Source: CAD feature listing. Evaluate the final solid. Frame: model axes, mm. Give positions to 0.01 mm unless a question says otherwise; leave off trailing zeros. Put each result on its own line as item: value. Start each with the question number.
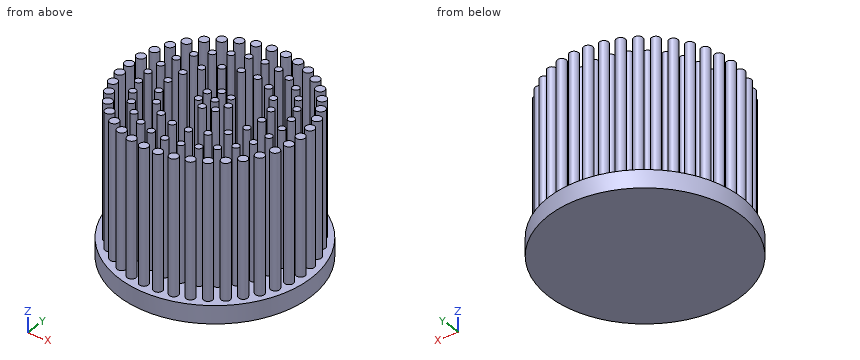
```python
from build123d import *

# Parameters (mm, degrees)
F2_R     = 43
F3_DEPTH = 8
F4_R     = 1.5
F4_R_2   = 2
F5_DEPTH = 60


with BuildPart() as f3:
    # F2 (on Top) → F3 (new body)
    with BuildSketch(Plane.XY):
        Circle(F2_R)
    extrude(amount=F3_DEPTH)

    # F4 (on face) → F5 (join)
    with BuildSketch(Plane.XY.offset(8)):
        Circle(F4_R)
        with Locations((6, 0)):
            Circle(F4_R)
        with Locations((21, 0)):
            Circle(F4_R)
        with Locations((38.41, 0)):
            Circle(F4_R_2)
        with Locations((3.7409388112, 4.6909888948)):
            Circle(F4_R)
        with Locations((-1.3351256037, 5.8495674731)):
            Circle(F4_R)
        with Locations((-5.4058132074, 2.6033024347)):
            Circle(F4_R)
        with Locations((-5.4058132074, -2.6033024347)):
            Circle(F4_R)
        with Locations((-1.3351256037, -5.8495674731)):
            Circle(F4_R)
        with Locations((3.7409388112, -4.6909888948)):
            Circle(F4_R)
        with Locations((19.7335450365, 7.1824230098)):
            Circle(F4_R)
        with Locations((16.0869333055, 13.4985398034)):
            Circle(F4_R)
        with Locations((10.5, 18.1865334795)):
            Circle(F4_R)
        with Locations((3.646611731, 20.6809628133)):
            Circle(F4_R)
        with Locations((-3.646611731, 20.6809628133)):
            Circle(F4_R)
        with Locations((-10.5, 18.1865334795)):
            Circle(F4_R)
        with Locations((-16.0869333055, 13.4985398034)):
            Circle(F4_R)
        with Locations((-19.7335450365, 7.1824230098)):
            Circle(F4_R)
        with Locations((-21, 0)):
            Circle(F4_R)
        with Locations((-19.7335450365, -7.1824230098)):
            Circle(F4_R)
        with Locations((-16.0869333055, -13.4985398034)):
            Circle(F4_R)
        with Locations((-10.5, -18.1865334795)):
            Circle(F4_R)
        with Locations((-3.646611731, -20.6809628133)):
            Circle(F4_R)
        with Locations((3.646611731, -20.6809628133)):
            Circle(F4_R)
        with Locations((10.5, -18.1865334795)):
            Circle(F4_R)
        with Locations((16.0869333055, -13.4985398034)):
            Circle(F4_R)
        with Locations((19.7335450365, -7.1824230098)):
            Circle(F4_R)
        with Locations((30, 0)):
            Circle(F4_R)
        with Locations((29.2478373655, 6.6756280187)):
            Circle(F4_R)
        with Locations((27.0290660371, 13.0165121735)):
            Circle(F4_R)
        with Locations((23.454944474, 18.7046940558)):
            Circle(F4_R)
        with Locations((18.7046940558, 23.454944474)):
            Circle(F4_R)
        with Locations((13.0165121735, 27.0290660371)):
            Circle(F4_R)
        with Locations((6.6756280187, 29.2478373655)):
            Circle(F4_R)
        with Locations((0, 30)):
            Circle(F4_R)
        with Locations((-6.6756280187, 29.2478373655)):
            Circle(F4_R)
        with Locations((-13.0165121735, 27.0290660371)):
            Circle(F4_R)
        with Locations((-18.7046940558, 23.454944474)):
            Circle(F4_R)
        with Locations((-23.454944474, 18.7046940558)):
            Circle(F4_R)
        with Locations((-27.0290660371, 13.0165121735)):
            Circle(F4_R)
        with Locations((-29.2478373655, 6.6756280187)):
            Circle(F4_R)
        with Locations((-30, 0)):
            Circle(F4_R)
        with Locations((-29.2478373655, -6.6756280187)):
            Circle(F4_R)
        with Locations((-27.0290660371, -13.0165121735)):
            Circle(F4_R)
        with Locations((-23.454944474, -18.7046940558)):
            Circle(F4_R)
        with Locations((-18.7046940558, -23.454944474)):
            Circle(F4_R)
        with Locations((-13.0165121735, -27.0290660371)):
            Circle(F4_R)
        with Locations((-6.6756280187, -29.2478373655)):
            Circle(F4_R)
        with Locations((0, -30)):
            Circle(F4_R)
        with Locations((6.6756280187, -29.2478373655)):
            Circle(F4_R)
        with Locations((13.0165121735, -27.0290660371)):
            Circle(F4_R)
        with Locations((18.7046940558, -23.454944474)):
            Circle(F4_R)
        with Locations((23.454944474, -18.7046940558)):
            Circle(F4_R)
        with Locations((27.0290660371, -13.0165121735)):
            Circle(F4_R)
        with Locations((29.2478373655, -6.6756280187)):
            Circle(F4_R)
        with Locations((37.8861376637, 6.3220782127)):
            Circle(F4_R_2)
        with Locations((36.3288402537, 12.4717066122)):
            Circle(F4_R_2)
        with Locations((33.7805867838, 18.2811393666)):
            Circle(F4_R_2)
        with Locations((30.3108869659, 23.5919102944)):
            Circle(F4_R_2)
        with Locations((26.0143851661, 28.259155409)):
            Circle(F4_R_2)
        with Locations((21.0082787535, 32.1555644301)):
            Circle(F4_R_2)
        with Locations((15.4291212609, 35.1748534768)):
            Circle(F4_R_2)
        with Locations((9.4290975611, 37.2346642147)):
            Circle(F4_R_2)
        with Locations((3.1718726596, 38.2788103764)):
            Circle(F4_R_2)
        with Locations((-3.1718726596, 38.2788103764)):
            Circle(F4_R_2)
        with Locations((-9.4290975611, 37.2346642147)):
            Circle(F4_R_2)
        with Locations((-15.4291212609, 35.1748534768)):
            Circle(F4_R_2)
        with Locations((-21.0082787535, 32.1555644301)):
            Circle(F4_R_2)
        with Locations((-26.0143851661, 28.259155409)):
            Circle(F4_R_2)
        with Locations((-30.3108869659, 23.5919102944)):
            Circle(F4_R_2)
        with Locations((-33.7805867838, 18.2811393666)):
            Circle(F4_R_2)
        with Locations((-36.3288402537, 12.4717066122)):
            Circle(F4_R_2)
        with Locations((-37.8861376637, 6.3220782127)):
            Circle(F4_R_2)
        with Locations((-38.41, 0)):
            Circle(F4_R_2)
        with Locations((-37.8861376637, -6.3220782127)):
            Circle(F4_R_2)
        with Locations((-36.3288402537, -12.4717066122)):
            Circle(F4_R_2)
        with Locations((-33.7805867838, -18.2811393666)):
            Circle(F4_R_2)
        with Locations((-30.3108869659, -23.5919102944)):
            Circle(F4_R_2)
        with Locations((-26.0143851661, -28.259155409)):
            Circle(F4_R_2)
        with Locations((-21.0082787535, -32.1555644301)):
            Circle(F4_R_2)
        with Locations((-15.4291212609, -35.1748534768)):
            Circle(F4_R_2)
        with Locations((-9.4290975611, -37.2346642147)):
            Circle(F4_R_2)
        with Locations((-3.1718726596, -38.2788103764)):
            Circle(F4_R_2)
        with Locations((3.1718726596, -38.2788103764)):
            Circle(F4_R_2)
        with Locations((9.4290975611, -37.2346642147)):
            Circle(F4_R_2)
        with Locations((15.4291212609, -35.1748534768)):
            Circle(F4_R_2)
        with Locations((21.0082787535, -32.1555644301)):
            Circle(F4_R_2)
        with Locations((26.0143851661, -28.259155409)):
            Circle(F4_R_2)
        with Locations((30.3108869659, -23.5919102944)):
            Circle(F4_R_2)
        with Locations((33.7805867838, -18.2811393666)):
            Circle(F4_R_2)
        with Locations((36.3288402537, -12.4717066122)):
            Circle(F4_R_2)
        with Locations((37.8861376637, -6.3220782127)):
            Circle(F4_R_2)
    extrude(amount=F5_DEPTH)


solid = f3.part
```
1. Contact query for flat-ended pins moving along their axis: pin 1 (8 mm diameter, centred on x = 32.5, z = 33, fed in from -Y); pin 2 (2 mm diameter, centred on x = -28, y = -34, fed in from +Z); pin 3 (6 mm diameter, centred on y = -32, z = 27.5, fed in from +X); pin 4 (6 mm diameter, centred on y = 18.5, z = 25, fed in from -X). Output: stop coordinate, or through.
2. Section A-A, the plane z = 25.5. State how many separate pieces and enclosed holes the cut face has, plus the area to 3 significant figures.
3. Ray query, line 1 (Y direction, x = -3.5, z = 54); line 2 (X direction, y = 28, z = 46.5); line 3 (X direction, y = -7.5, z = 57). Return the intervals inside material, ascending.
Results found:
1. pin 1: y = -25.59
1. pin 2: through
1. pin 3: x = 27.87
1. pin 4: x = -35.78
2. separate pieces: 92
2. enclosed holes: 0
2. area: 859 mm²
3. line 1: -40.25 to -36.31, -22.17 to -19.19, 19.19 to 22.17, 36.31 to 40.25
3. line 2: -28 to -24.03, -14.16 to -11.87, -7.51 to -5.84, 5.84 to 7.51, 11.87 to 14.16, 24.03 to 28
3. line 3: -39.5 to -36.27, -30.5 to -27.99, -21.2 to -18.27, 18.27 to 21.2, 27.99 to 30.5, 36.27 to 39.5
